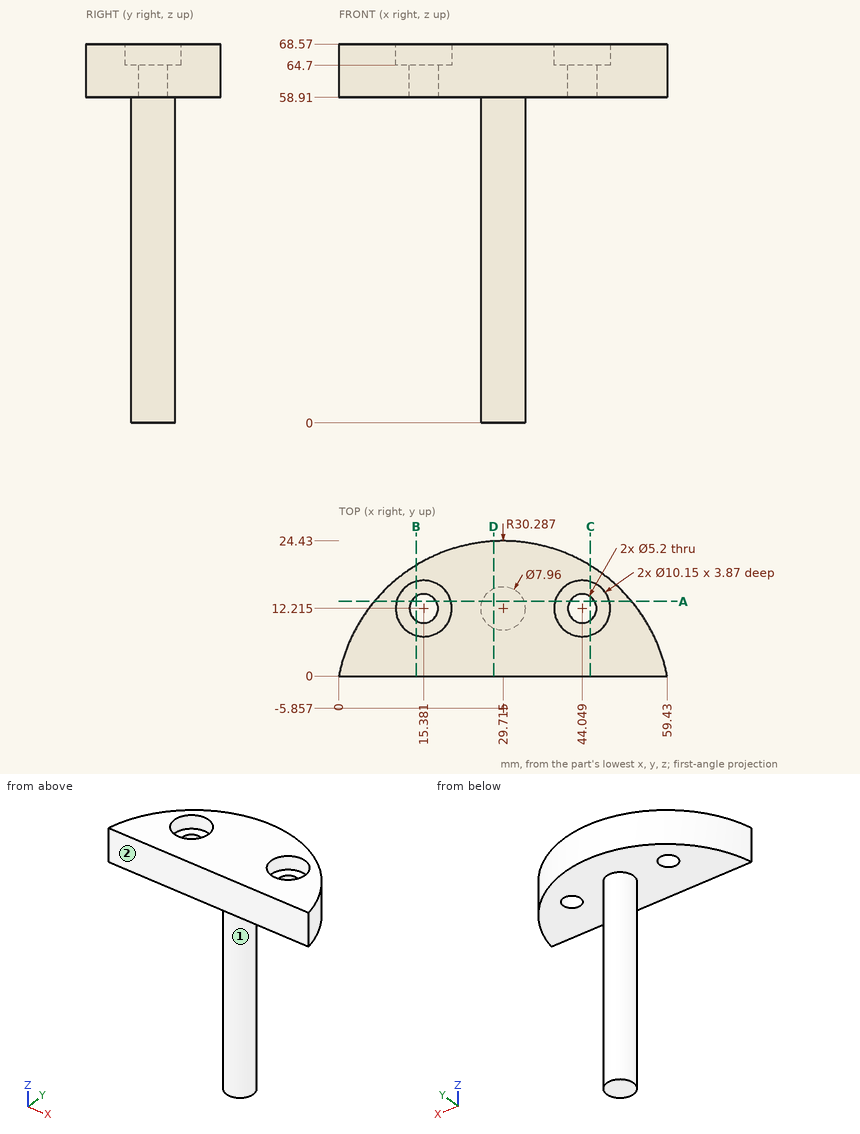
Check sheet for the drawn part. Datum: minimum x, y, z corner. Units: mm. A direction names the side the tool comes from. Round coordinates to 2 decimals unless told otherwise and drop trailing zeros. Loops run counter-clockwise (first coordinate to the right, second up) from the corner with the lowest first, then second, coordinate; pieces in that order, holes last. Notation, with made-up numbers: M -32.75,38.5 L 17.25,38.5 A36 cw 17.25,72.5 Z; hole C -8.5,21.5 d10. An arc over 180 degrees is marked long. One line per question, with ' | ' between items. Start each with the question number.
Item 1: Section check C-C (x = 45.5). Record the boundary of the cut face in (y, z).
Item 2: Set-up check for the marked faces 1 and 2: record each of +Z, -Z, +X, -X, +Y, -Y from which the full face is reachable in a straight line by a thin tool's end or side.
Item 3: Section check B-B (x = 14). Record the boundary of the cut face in (y, z).
Item 4: Section check D-D (x = 28). Record the boundary of the cut face in (y, z).
Item 5: Scan lines: probe 1 along Z at (x, y) = (31, 23); probe 2 along Y at (x, z) = (11.5, 59); probe 3 along X at (y, z) = (9, 33). Record each from-to range of solid material in increasing order.
Item 6: Section check A-A (y = 13.5). Record the boundary of the cut face in (x, z).
Item 7: Gauge pin test, flat ends, axial feed: pin 1 Ø11 at (x, y) = (14, 12.5) entering from +Z; pin 2 Ø9 at (x, y) = (44.05, 12.22) entering from +Z; pin 3 Ø1 at (y, z) = (6.5, 21.5) entering from -X; pin 4 Ø5 at (y, z) = (6.5, 34.5) entering from +X. Record the tip position at first contact, or that the pin passes through.
Worked out:
1) outline: M 0,58.91 L 10.06,58.91 L 10.06,64.7 L 7.35,64.7 L 7.35,68.57 L 0,68.57 Z; M 14.37,58.91 L 19.99,58.91 L 19.99,68.57 L 17.08,68.57 L 17.08,64.7 L 14.37,64.7 Z
2) face 1: -Z | face 2: +Z, -Z, +X, -X, -Y
3) outline: M 0,58.91 L 10.01,58.91 L 10.01,64.7 L 7.33,64.7 L 7.33,68.57 L 0,68.57 Z; M 14.42,58.91 L 20.03,58.91 L 20.03,68.57 L 17.1,68.57 L 17.1,64.7 L 14.42,64.7 Z
4) outline: M 0,58.91 L 8.62,58.91 L 8.62,0 L 15.81,0 L 15.81,58.91 L 24.38,58.91 L 24.38,68.57 L 0,68.57 Z
5) probe 1: 58.91 to 68.57 | probe 2: 0 to 18.34 | probe 3: 27.37 to 32.06
6) outline: M 6.42,58.91 L 13.12,58.91 L 13.12,64.7 L 10.47,64.7 L 10.47,68.57 L 6.42,68.57 Z; M 17.64,58.91 L 25.95,58.91 L 25.95,0 L 33.48,0 L 33.48,58.91 L 41.79,58.91 L 41.79,64.7 L 39.14,64.7 L 39.14,68.57 L 20.29,68.57 L 20.29,64.7 L 17.64,64.7 Z; M 46.31,58.91 L 53.01,58.91 L 53.01,68.57 L 48.96,68.57 L 48.96,64.7 L 46.31,64.7 Z
7) pin 1: z = 68.57 | pin 2: z = 64.7 | pin 3: through | pin 4: x = 32.06
